Can you work these out from the model? Positions are in its coordinate system, mm. Face numbers are marked on the shaded views. A direction names the side the tool comes from. Give positions to 0.01 mm unless a question says otherwise; leave off trailing zeros. Order: outer loops, then holes, each group sorted by start corner. A loop starts at its lowest first (then second) coordinate and runs counter-clockwise, first axis right, second up. Notation, with made-up numbers: (-24, -40) - (9, -40) arc R7 cw to (9, -31) - close; hole circle Ø1 at (-11, 38.25). An arc over 180 degrees is marked (long way). One line per question, with ' | ' between items.
```python
from build123d import *

# Parameters (mm, degrees)
F0_W     = 15
F0_H     = 15
F1_DEPTH = 20
F2_DEPTH = 40
F4_DEPTH = 20
F6_DEPTH = 20


with BuildPart() as f1:
    # F0 (on Right) → F1 (new body)
    with BuildSketch(Plane.YZ):
        with Locations((7.5, 7.5)):
            Rectangle(F0_W, F0_H)
        with Locations((22.5, 7.5)):
            Rectangle(F0_W, F0_H)
        with Locations((7.5, 22.5)):
            Rectangle(F0_W, F0_H)
        with Locations((22.5, 22.5)):
            Rectangle(F0_W, F0_H)
    extrude(amount=F1_DEPTH)

    # F0 (on Right) → F2 (join)
    with BuildSketch(Plane.YZ):
        with Locations((22.5, 7.5)):
            Rectangle(F0_W, F0_H)
        with Locations((22.5, 22.5)):
            Rectangle(F0_W, F0_H)
        with Locations((7.5, 22.5)):
            Rectangle(F0_W, F0_H)
    extrude(amount=F2_DEPTH)

    # F3 (on face) → F4 (cut)
    with BuildSketch(Plane.YZ.offset(40)):
        Polygon((30, 30), (15, 30), (30, 15), align=None)
    extrude(amount=-F4_DEPTH, mode=Mode.SUBTRACT)

    # F5 (on face) → F6 (cut)
    with BuildSketch(Plane.YZ.offset(40)):
        Polygon((30, 0), (15, 15), (15, 0), align=None)
    extrude(amount=-F6_DEPTH, mode=Mode.SUBTRACT)


solid = f1.part
```
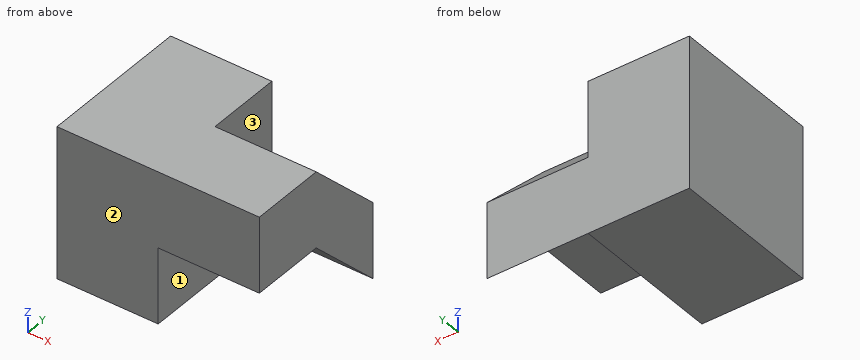
(1) Imagine slicing it at A-A (z = 20.5). List the corners of the cut face in (x, y) for me.
Answer below:
outline: (0, 0) - (40, 0) - (40, 24.5) - (20, 24.5) - (20, 30) - (0, 30) - close
(2) Imagine slicing it at B-B (x = 26.5). List the corners of the cut face in (y, z) for me, and give its area (3 significant figures).
Answer below:
outline: (0, 15) - (15, 15) - (30, 0) - (30, 15) - (15, 30) - (0, 30) - close | area: 450 mm^2
(3) Will these pins go through, and if not, where does the flat tip stop? pin 1 (16.5 mm diameter, centred on x = 27, y = 8, fed in from -Z); pin 2 (6 mm diameter, centred on x = 25.5, z = 10, fed in from -Y); pin 3 (6 mm diameter, centred on x = 24.5, y = 14.5, fed in from -Z); pin 4 (1 mm diameter, centred on x = 35.5, y = 23.5, fed in from +Z).
Answer below:
pin 1: z = 0 | pin 2: y = 17 | pin 3: z = 12.5 | pin 4: z = 22
(4) If I drill on line 1 (Z direction, x = 34, y = 11); line 2 (X direction, y = 17, z = 5.5); line 3 (Y direction, x = 28.5, z = 4), over which ranges is the centre line in solid material (lowest first)?
Answer below:
line 1: 15 to 30 | line 2: 0 to 20 | line 3: 26 to 30
(5) On a 3-axis mill with a long thin cutter (end or side, diameter ignored), from which of +Z, -Z, +X, -X, +Y, -Y can I reach the whole of each face in a straight line? I mean the marked faces 1, 2 and 3. Say none if no direction works.
Answer below:
face 1: -Z, +X, -Y | face 2: +Z, -Z, +X, -X, -Y | face 3: +Z, +X, +Y
